```python
from build123d import *

# Parameters (mm, degrees)
SKETCH_1_W          = 240
SKETCH_1_H          = 180
SKETCH_1_R          = 51
SKETCH_1_R_2        = 1.6
SKETCH_1_R_3        = 2.1
SKETCH_1_R_4        = 1.25
EXTRUDE_1_DEPTH     = 10
CUT_EXTRUDE_1_DEPTH = 11
SKETCH_3_R          = 2.6
SKETCH_3_W          = 240
SKETCH_3_H          = 1
CUT_EXTRUDE_2_DEPTH = 11
CUT_EXTRUDE_3_DEPTH = 11
FILLET_1_R          = 10
CUT_EXTRUDE_4_DEPTH = 11
CHAMFER_1_SIZE      = 1.5


with BuildPart() as part:
    # 草图1 → 凸台-拉伸1 (new body)
    with BuildSketch(Plane(origin=(0, 0, 0), x_dir=(1, 0, 0), z_dir=(0, 1, 0))):
        Rectangle(SKETCH_1_W, SKETCH_1_H)
        Circle(SKETCH_1_R, mode=Mode.SUBTRACT)
        with Locations((0, 56)):
            Circle(SKETCH_1_R_2, mode=Mode.SUBTRACT)
        with Locations((28, 48.497422612)):
            Circle(SKETCH_1_R_2, mode=Mode.SUBTRACT)
        with Locations((48.497422612, 28)):
            Circle(SKETCH_1_R_2, mode=Mode.SUBTRACT)
        with Locations((56, 0)):
            Circle(SKETCH_1_R_2, mode=Mode.SUBTRACT)
        with Locations((48.497422612, -28)):
            Circle(SKETCH_1_R_2, mode=Mode.SUBTRACT)
        with Locations((28, -48.497422612)):
            Circle(SKETCH_1_R_2, mode=Mode.SUBTRACT)
        with Locations((0, -56)):
            Circle(SKETCH_1_R_2, mode=Mode.SUBTRACT)
        with Locations((-28, -48.497422612)):
            Circle(SKETCH_1_R_2, mode=Mode.SUBTRACT)
        with Locations((-48.497422612, -28)):
            Circle(SKETCH_1_R_2, mode=Mode.SUBTRACT)
        with Locations((-56, 0)):
            Circle(SKETCH_1_R_2, mode=Mode.SUBTRACT)
        with Locations((-48.497422612, 28)):
            Circle(SKETCH_1_R_2, mode=Mode.SUBTRACT)
        with Locations((-28, 48.497422612)):
            Circle(SKETCH_1_R_2, mode=Mode.SUBTRACT)
        with Locations((-70, 85)):
            Circle(SKETCH_1_R_3, mode=Mode.SUBTRACT)
        with Locations((-50, 85)):
            Circle(SKETCH_1_R_3, mode=Mode.SUBTRACT)
        with Locations((-70, 65)):
            Circle(SKETCH_1_R_3, mode=Mode.SUBTRACT)
        with Locations((-50, 65)):
            Circle(SKETCH_1_R_3, mode=Mode.SUBTRACT)
        with Locations((50, 85)):
            Circle(SKETCH_1_R_3, mode=Mode.SUBTRACT)
        with Locations((50, 65)):
            Circle(SKETCH_1_R_3, mode=Mode.SUBTRACT)
        with Locations((70, 65)):
            Circle(SKETCH_1_R_3, mode=Mode.SUBTRACT)
        with Locations((70, 85)):
            Circle(SKETCH_1_R_3, mode=Mode.SUBTRACT)
        with Locations((70, -85)):
            Circle(SKETCH_1_R_3, mode=Mode.SUBTRACT)
        with Locations((70, -65)):
            Circle(SKETCH_1_R_3, mode=Mode.SUBTRACT)
        with Locations((50, -65)):
            Circle(SKETCH_1_R_3, mode=Mode.SUBTRACT)
        with Locations((50, -85)):
            Circle(SKETCH_1_R_3, mode=Mode.SUBTRACT)
        with Locations((-50, -65)):
            Circle(SKETCH_1_R_3, mode=Mode.SUBTRACT)
        with Locations((-70, -65)):
            Circle(SKETCH_1_R_3, mode=Mode.SUBTRACT)
        with Locations((-50, -85)):
            Circle(SKETCH_1_R_3, mode=Mode.SUBTRACT)
        with Locations((-70, -85)):
            Circle(SKETCH_1_R_3, mode=Mode.SUBTRACT)
        with Locations((112, 10)):
            Circle(SKETCH_1_R_4, mode=Mode.SUBTRACT)
        with Locations((112, 30)):
            Circle(SKETCH_1_R_4, mode=Mode.SUBTRACT)
        with Locations((112, -30)):
            Circle(SKETCH_1_R_4, mode=Mode.SUBTRACT)
        with Locations((112, -10)):
            Circle(SKETCH_1_R_4, mode=Mode.SUBTRACT)
        with Locations((-112, -30)):
            Circle(SKETCH_1_R_4, mode=Mode.SUBTRACT)
        with Locations((-112, -10)):
            Circle(SKETCH_1_R_4, mode=Mode.SUBTRACT)
        with Locations((-112, 30)):
            Circle(SKETCH_1_R_4, mode=Mode.SUBTRACT)
        with Locations((-112, 10)):
            Circle(SKETCH_1_R_4, mode=Mode.SUBTRACT)
    extrude(amount=EXTRUDE_1_DEPTH)

    # 草图2 → 切除-拉伸1 (cut, through all)
    with BuildSketch(Plane(origin=(0, 10, 0), x_dir=(1, 0, 0), z_dir=(0, 1, 0))):
        Polygon((-120, 57.5), (-110, 47.5), (-110, -47.5), (-120, -57.5), align=None)
        Polygon((110, -47.5), (120, -57.5), (120, 57.5), (110, 47.5), align=None)
    extrude(amount=-CUT_EXTRUDE_1_DEPTH, mode=Mode.SUBTRACT)

    # 草图3 → 切除-拉伸2 (cut, through all)
    with BuildSketch(Plane(origin=(0, 10, 0), x_dir=(1, 0, 0), z_dir=(0, 1, 0))):
        with Locations((-30, 83)):
            Circle(SKETCH_3_R)
        with Locations((0, 83)):
            Circle(SKETCH_3_R)
        with Locations((30, 83)):
            Circle(SKETCH_3_R)
        with Locations((30, -83)):
            Circle(SKETCH_3_R)
        with Locations((0, -83)):
            Circle(SKETCH_3_R)
        with Locations((-30, -83)):
            Circle(SKETCH_3_R)
        with Locations((0, 89.5)):
            Rectangle(SKETCH_3_W, SKETCH_3_H)
        with Locations((0, -89.5)):
            Rectangle(SKETCH_3_W, SKETCH_3_H)
    extrude(amount=-CUT_EXTRUDE_2_DEPTH, mode=Mode.SUBTRACT)

    # 草图4 → 切除-拉伸3 (cut, through all)
    with BuildSketch(Plane(origin=(0, 10, 0), x_dir=(1, 0, 0), z_dir=(0, 1, 0))):
        with BuildLine():
            Line((-38.483126456, 89), (-62.209561842, 22.044736684))
            ThreePointArc((-62.209561842, 22.044736684), (-66, 0), (-62.209561842, -22.044736684))
            Line((-62.209561842, -22.044736684), (-38.483126456, -89))
            Line((-38.483126456, -89), (-120, -89))
            Line((-120, -89), (-120, 89))
            Line((-120, 89), (-38.483126456, 89))
        make_face()
        with BuildLine():
            Line((120, -89), (120, 89))
            Line((120, 89), (38.483126456, 89))
            Line((38.483126456, 89), (62.209561842, 22.044736684))
            ThreePointArc((62.209561842, 22.044736684), (66, 0), (62.209561842, -22.044736684))
            Line((62.209561842, -22.044736684), (38.483126456, -89))
            Line((38.483126456, -89), (120, -89))
        make_face()
    extrude(amount=-CUT_EXTRUDE_3_DEPTH, mode=Mode.SUBTRACT)

    # 圆角1
    fillet_1_edges = [part.edges().sort_by_distance(p)[0] for p in [
        (-38.483126456, 5, -89),
        (-38.483126456, 5, 89),
        (38.483126456, 5, 89),
        (38.483126456, 5, -89),
    ]]
    fillet(fillet_1_edges, radius=FILLET_1_R)

    # 草图7 → 切除-拉伸4 (cut, through all)
    with BuildSketch(Plane(origin=(0, 10, 0), x_dir=(1, 0, 0), z_dir=(0, 1, 0))):
        with BuildLine():
            Line((-9, 76.5), (-28.061793108, 76.5))
            ThreePointArc((-28.061793108, 76.5), (-29.792963167, 75.950112289), (-30.889500465, 74.502033486))
            Line((-30.889500465, 74.502033486), (-35.375296407, 61.843256739))
            ThreePointArc((-35.375296407, 61.843256739), (-34.503237981, 58.566264515), (-31.132476483, 58.195952677))
            ThreePointArc((-31.132476483, 58.195952677), (-20.197656361, 62.833547389), (-8.608695652, 65.436154832))
            ThreePointArc((-8.608695652, 65.436154832), (-6.744571765, 66.432384086), (-6, 68.410525506))
            Line((-6, 68.410525506), (-6, 73.5))
            ThreePointArc((-6, 73.5), (-6.878679656, 75.621320344), (-9, 76.5))
        make_face()
        with BuildLine():
            Line((9, 76.5), (28.061793108, 76.5))
            ThreePointArc((28.061793108, 76.5), (29.792963167, 75.950112289), (30.889500465, 74.502033486))
            Line((30.889500465, 74.502033486), (35.375296407, 61.843256739))
            ThreePointArc((35.375296407, 61.843256739), (34.503237981, 58.566264515), (31.132476483, 58.195952677))
            ThreePointArc((31.132476483, 58.195952677), (20.197656361, 62.833547389), (8.608695652, 65.436154832))
            ThreePointArc((8.608695652, 65.436154832), (6.744571765, 66.432384086), (6, 68.410525506))
            Line((6, 68.410525506), (6, 73.5))
            ThreePointArc((6, 73.5), (6.878679656, 75.621320344), (9, 76.5))
        make_face()
        with BuildLine():
            Line((6, -73.5), (6, -68.410525506))
            ThreePointArc((6, -68.410525506), (6.744571765, -66.432384086), (8.608695652, -65.436154832))
            ThreePointArc((8.608695652, -65.436154832), (20.197656361, -62.833547389), (31.132476483, -58.195952677))
            ThreePointArc((31.132476483, -58.195952677), (34.503237981, -58.566264515), (35.375296407, -61.843256739))
            Line((35.375296407, -61.843256739), (30.889500465, -74.502033486))
            ThreePointArc((30.889500465, -74.502033486), (29.792963167, -75.950112289), (28.061793108, -76.5))
            Line((28.061793108, -76.5), (9, -76.5))
            ThreePointArc((9, -76.5), (6.878679656, -75.621320344), (6, -73.5))
        make_face()
        with BuildLine():
            Line((-9, -76.5), (-28.061793108, -76.5))
            ThreePointArc((-28.061793108, -76.5), (-29.792963167, -75.950112289), (-30.889500465, -74.502033486))
            Line((-30.889500465, -74.502033486), (-35.375296407, -61.843256739))
            ThreePointArc((-35.375296407, -61.843256739), (-34.503237981, -58.566264515), (-31.132476483, -58.195952677))
            ThreePointArc((-31.132476483, -58.195952677), (-20.197656361, -62.833547389), (-8.608695652, -65.436154832))
            ThreePointArc((-8.608695652, -65.436154832), (-6.744571765, -66.432384086), (-6, -68.410525506))
            Line((-6, -68.410525506), (-6, -73.5))
            ThreePointArc((-6, -73.5), (-6.878679656, -75.621320344), (-9, -76.5))
        make_face()
    extrude(amount=-CUT_EXTRUDE_4_DEPTH, mode=Mode.SUBTRACT)

    # 倒角1
    chamfer_1_edges = [part.edges().sort_by_distance(p)[0] for p in [
        (-1.6, 10, -56),
        (26.4, 10, -48.497422612),
        (26.4, 10, 48.497422612),
        (-1.6, 10, 56),
        (-29.6, 10, 48.497422612),
        (-29.6, 10, -48.497422612),
    ]]
    chamfer(chamfer_1_edges, length=CHAMFER_1_SIZE)


solid = part.part
```
The listing builds one solid part. Answer for the finished solid, in the listing's coordinates (mm). A direction names the side the tool comes from. Give positions to 0.01 mm unless a question says otherwise; leave off trailing zeros. Write each loop counter-clockwise with the first axis right and the second up, starting at its lowest first coordinate (ties: lowest second). Pieces come first, ordered by that corner, then holes. Notation, with made-up numbers: (80, -11.75) - (94, -11.75) arc R10 cw to (94, -4.75) - close; hole circle Ø5 at (53, 74). An arc over 180 degrees is marked (long way). Use one line per item in the form item = value. Start each with the question number.
1) Flat-ended cylindrical pins translate along their axes: pin 1 Ø3 at (x, z) = (-30, 83) entering from +Y; pin 2 Ø6 at (y, z) = (6.5, 27.5) entering from -X; pin 3 Ø5 at (y, z) = (5, -27.5) entering from -X; pin 4 Ø5 at (y, z) = (1.5, -4.5) entering from -X. Find the tip coordinate at first contact, or state that the pin passes through.
2) Find section C-C on x = -43. Determine the outline of the cut face in (y, z).
3) Consider line 1 along Z through (x, y) = (0, 5.5); line 2 along X through (y, z) = (1.5, -70.5); line 3 along X through (y, z) = (2.5, -28). Determine where each line is inside the solid, lowest interval first. Write a range as from..to.
4) Find section B-B on x = -11.5. Determine the outline of the cut face in (y, z), plus the area to 3 significant figures.
5) Find section A-A on z = -43.5. Determine the outline of the cut face in (x, y).
6) A tool of negligible diameter and unlimited length cuts with its end or side. For faces 1 (the face through (-20.36, 5.07, -62.78)), 2 (the face through (51.38, 5.07, -52.61)), from which of +Z, -Z, +X, -X, +Y, -Y can it reach the whole face along a straight path? Write none if from no direction.
7) The mould has two halves that part along X. Classify faces 3 (the face through (-33.1, 5.07, -68.26)), 4 (the face through (37.117, 4.93, -87.216)), 5 (the face through (-51.676, 5.07, 51.77)): pulls with the +X half, pulls with the -X half, needs draft (parallel to the pull), parting line crosses it, or undercut.
8) Find section D-D on x = 20. Determine the outline of the cut face in (y, z).
Geometry results:
q1.pin_1 = through
q1.pin_2 = -61.34
q1.pin_3 = -61.16
q1.pin_4 = -65.97
q2.outline = (0, -76.25) - (10, -76.25) - (10, -27.42) - (0, -27.42) - close; (0, 27.42) - (10, 27.42) - (10, 76.25) - (0, 76.25) - close
q3.line_1 = -89..-85.6, -80.4..-57.6, -54.4..-51, 51..54.4, 57.6..80.4, 85.6..89
q3.line_2 = -45.04..-32.31, -6..6, 32.31..45.04
q3.line_3 = -60.1..-50.1, -46.9..-42.63, 42.63..46.9, 50.1..60.1
q4.outline = (0, -89) - (10, -89) - (10, -76.5) - (0, -76.5) - close; (0, -64.99) - (10, -64.99) - (10, -49.69) - (0, -49.69) - close; (0, 49.69) - (10, 49.69) - (10, 64.99) - (0, 64.99) - close; (0, 76.5) - (10, 76.5) - (10, 89) - (0, 89) - close
q4.area = 556 mm2
q5.outline = (-54.61, 0) - (-26.62, 0) - (-26.62, 10) - (-54.61, 10) - close; (26.62, 0) - (54.61, 0) - (54.61, 10) - (26.62, 10) - close
q6.face_1 = +Y, -Y
q6.face_2 = -Z, +X, +Y, -Y
q7.face_3 = undercut
q7.face_4 = pulls with the +X half
q7.face_5 = pulls with the -X half
q8.outline = (0, -89) - (10, -89) - (10, -76.5) - (0, -76.5) - close; (0, -62.9) - (10, -62.9) - (10, -46.91) - (0, -46.91) - close; (0, 46.91) - (10, 46.91) - (10, 62.9) - (0, 62.9) - close; (0, 76.5) - (10, 76.5) - (10, 89) - (0, 89) - close
